```python
from build123d import *

# Parameters (mm, degrees)
CUT_EXTRUDE1_DEPTH      = 113.222992297
CUT_EXTRUDE1_DEPTH_BACK = 113.222992297
SKETCH2_R               = 2.5
CUT_EXTRUDE2_DEPTH      = 113.222992405
CUT_EXTRUDE2_DEPTH_BACK = 113.222992405
SKETCH4_R               = 2.5


with BuildPart() as part:
    # Sketch1 → Revolve1 (revolve)
    with BuildSketch(Plane.XY):
        Polygon((0, 0), (0, 4), (-10, 4), (-10, 5), (-37, 5), (-37, 4.6), (-37.66, 4.6), (-37.66, 5), (-77.34, 5), (-77.34, 4.6), (-78, 4.6), (-78, 5), (-84, 5), (-84, 4.6), (-84.66, 4.6), (-84.66, 5), (-87.34, 5), (-87.34, 4.6), (-88, 4.6), (-88, 5), (-112, 5), (-112, 0), align=None)
    revolve(axis=Axis((0, 0, 0), (-1, 0, 0)))

    # Sketch2 → Cut-Extrude1 (cut, two sides: drawn at the far end of the back side and taken through both)
    with BuildSketch(Plane(origin=(0, 0, 0), x_dir=(1, 0, 0), z_dir=(0, 1, 0)).offset(-CUT_EXTRUDE1_DEPTH_BACK)):
        with Locations((-103, 0)):
            Circle(SKETCH2_R)
    extrude(amount=CUT_EXTRUDE1_DEPTH + CUT_EXTRUDE1_DEPTH_BACK, mode=Mode.SUBTRACT)

    # Sketch4 → Cut-Extrude2 (cut, two sides: drawn at the far end of the back side and taken through both)
    with BuildSketch(Plane.XY.offset(-CUT_EXTRUDE2_DEPTH_BACK)):
        with Locations((-94, 0)):
            Circle(SKETCH4_R)
    extrude(amount=CUT_EXTRUDE2_DEPTH + CUT_EXTRUDE2_DEPTH_BACK, mode=Mode.SUBTRACT)


solid = part.part
```
Verification items for the finished model (mm, model axes). A direction names the side the tool comes from. Coordinates: 2 decimals unless noted, no trailing zeros. Loops run counter-clockwise (first coordinate to the right, second up) from the corner with the lowest first, then second, coordinate; pieces in that order, holes last. Notation, with made-up numbers: (-17, -22) - (-10, -22) arc R25 ccw to (-10, 1) - close; hole circle Ø10 at (37.25, 8). An arc over 180 degrees is marked (long way). Put each result on its own line as item: value.
Item 1: Section check D-D (x = -94). Enter the section's corners in (y, z).
Conclusion:
outline: (-2.5, -4.33) - (-2.5, 4.33) arc R5 ccw to start; (2.5, -4.33) arc R5 ccw to (2.5, 4.33) - close
Item 2: Set-up check for faces 1 (the face through (0, 0, 0)), 2 (the face through (-37.33, -3.65, 2.8)): record each of +Z, -Z, +X, -X, +Y, -Y from which the full face is reachable in a straight line by a thin tool's end or side.
Conclusion:
face 1: +Z, -Z, +X, +Y, -Y
face 2: none
Item 3: Draft check along X on faces 3 (the face through (-77.67, -3.65, 2.8)), 4 (the face through (-112, 0, 0)), 5 (the face through (-5.07, -0.867, 3.905)), 6 (the face through (-87.67, -3.65, 2.8)). Enter one of: pulls with the +X half, pulls with the -X half, needs draft (parallel to the pull), parting line crosses it, or undercut.
Conclusion:
face 3: undercut
face 4: pulls with the -X half
face 5: needs draft
face 6: undercut
Item 4: Section check C-C (x = -65). Enter the section's corners in (y, z), then the cut area to 3 significant figures.
Conclusion:
outline: circle Ø10 at (0, 0)
area: 78.5 mm2
Item 5: Section check A-A (z = 0). Give the number of separate pieces and of enclosed holes in the cut face, then the cut area to 3 significant figures.
Conclusion:
separate pieces: 2
enclosed holes: 1
area: 1,030 mm2
Item 6: Gauge pin test, flat ends, axial feed: pin 1 Ø1.5 at (x, z) = (-87, -3.5) entering from +Y; pin 2 Ø5 at (x, y) = (-57, 3) entering from +Z; pin 3 Ø4.5 at (x, y) = (-94, 0) entering from -Z; pin 4 Ø2 at (x, y) = (-50, -4) entering from +Z. Record the tip position at first contact, or that the pin passes through.
Conclusion:
pin 1: stops at y = 4.18
pin 2: stops at z = 4.97
pin 3: passes through
pin 4: stops at z = 4
Item 7: Scan lines: line 1 along X through (y, z) = (0, 3.25); line 2 along X through (y, z) = (-1.25, 0.25); line 3 along X through (y, z) = (2.75, 0). Record each from-to range of solid material in increasing order.
Conclusion:
line 1: x = -112 to -96.5, -91.5 to 0
line 2: x = -112 to -105.49, -100.51 to -96.17, -91.83 to 0
line 3: x = -112 to -105.5, -100.5 to 0
